The model under review builds one solid part; all positions refer to its coordinate system, in mm. A direction names the side the tool comes from. Round coordinates to 2 decimals unless told otherwise and drop trailing zeros. Order: outer loops, then holes, each group sorted by start corner. A loop starts at its lowest first (then second) coordinate and runs counter-clockwise, first axis right, second up.
Autodesk Fusion 360 part; units mm, degrees
sketch "Sketch1" plane through (0, 0, 0) normal (1, 0, 0) x (0, 0, -1)
  line L0 (-30.1, 40) -> (30.1, 40)
  line L1 (30.1, 40) -> (30.1, -40)
  line L2 (30.1, -40) -> (-30.1, -40)
  line L3 (-30.1, -40) -> (-30.1, 40)
  line L4 (-30.1, 40) -> (30.1, -40) construction
  line L5 (30.1, 40) -> (-30.1, -40) construction
  line L6 (-30.1, 40) -> (-65.1, 40)
  line L7 (-65.1, 40) -> (-65.1, -60)
  line L8 (-65.1, -60) -> (65.1, -60)
  line L9 (65.1, -60) -> (65.1, 40)
  line L10 (65.1, 40) -> (30.1, 40)
  dimension "d1" = 60.2
  dimension "d2" = 80
  dimension "d3" = 35
  dimension "d4" = 20
extrude "Extrude1" add sketch "Sketch1" along normal blind 30 contours L1 L2 L3 L6 L7 L8 L9 L10 makes body 1
sketch "Sketch2" plane through (0, 0, 0) normal (-1, 0, 0) x (0, 0, 1)
  line L0 (-30.1, 40) -> (-65.1, 40)
  line L1 (-65.1, 40) -> (-65.1, -60)
  line L2 (-65.1, -60) -> (65.1, -60)
  line L3 (65.1, -60) -> (65.1, 40)
  line L4 (65.1, 40) -> (30.1, 40)
  line L5 (30.1, 40) -> (30.1, -40)
  line L6 (30.1, -40) -> (-30.1, -40)
  line L7 (-30.1, -40) -> (-30.1, 40)
  line L8 (-47.6, 40) -> (-47.6, -60) construction
  circle A0 centre (-47.6, -0.3557) radius 10.5
  circle A1 centre (-47.6, -40.3557) radius 10.5
  line L9 (0, 0) -> (0, -40) construction
  circle A2 centre (-47.6, -0.3557) radius 4.25
  circle A3 centre (-47.6, -40.3557) radius 4.25
  circle A4 centre (47.6, -0.3557) radius 10.5
  circle A5 centre (47.6, -0.3557) radius 4.25
  circle A6 centre (47.6, -40.3557) radius 4.25
  circle A7 centre (47.6, -40.3557) radius 10.5
  dimension "d8" = 21
  dimension "d11" = 19.6443
  dimension "d12" = 8.5
  dimension "d13" = 8.5
  dimension "d14" = 40
chamfer "Chamfer2" distance 15 angle 45 2 edges at (15, 40, 65.1) (15, 40, -65.1) on bodies 1
chamfer "Chamfer1" distance 15 angle 45 2 edges at (30, -10, 65.1) (30, -10, -65.1) on bodies 1
extrude "Extrude2" cut sketch "Sketch2" against normal blind 60 contours A0 | A1 | A2 | A3 | A4 | A5 | A6 | A7 bodies 1
extrude "Extrude3" add sketch "Sketch2" against normal blind 20 contours A0 | A1 | A4 | A7 bodies 1
sketch "Sketch3" plane through (0, -40, 0) normal (0, 1, 0) x (-1, 0, 0)
  line L0 (0, -30.1) -> (0, 30.1)
  line L1 (0, 30.1) -> (-30, 30.1)
  line L2 (-30, 30.1) -> (-30, -30.1)
  line L3 (-30, -30.1) -> (0, -30.1)
  line L4 (0, 0) -> (-30, 0) construction
  line L5 (-15, 0) -> (-15, 15) construction
  circle A0 centre (-15, 15) radius 5
  circle A1 centre (-15, 15) radius 2.7
  circle A2 centre (-15, -15) radius 5
  circle A3 centre (-15, -15) radius 2.7
  dimension "d20" = 15
  dimension "d21" = 10
  dimension "d22" = 5.4
extrude "Extrude4" cut sketch "Sketch3" against normal blind 20 contours A0 | A1 | A2 | A3 bodies 1
extrude "Extrude5" add sketch "Sketch3" against normal blind 16 contours A0 | A2 bodies 1
sketch "Sketch4" plane through (0, 0, 30.1) normal (0, 0, -1) x (-1, 0, 0)
  line L0 (0, -40) -> (0, 40)
  line L1 (0, 40) -> (-30, 40)
  line L2 (-30, 40) -> (-30, -40)
  line L3 (-30, -40) -> (0, -40)
  line L4 (-15, 40) -> (-15, -40) construction
  circle A0 centre (-15, 25) radius 5
  circle A1 centre (-15, -20) radius 5
  circle A2 centre (-15, -20) radius 2.7
  circle A3 centre (-15, 25) radius 2.7
  dimension "d27" = 10
  dimension "d28" = 5.4
  dimension "d29" = 15
  dimension "d30" = 20
extrude "Extrude6" cut sketch "Sketch4" along normal blind 150 and the other way blind 65 contours A0 | A1 | A2 | A3 bodies 1
extrude "Extrude7" add sketch "Sketch4" against normal blind 18 contours A0 bodies 1
extrude "Extrude8" add sketch "Sketch4" against normal blind 7 contours A1 bodies 1
extrude "Extrude9" add sketch "Sketch4" along normal blind 18 from surface at 60.2 contours A0 bodies 1
extrude "Extrude10" add sketch "Sketch4" along normal blind 7 from surface at 60.2 contours A1 bodies 1
chamfer "Chamfer3" distance 0.4 angle 45 10 faces at (13.3333, -0.5675, 51.8447) (13.3333, -40.5675, 51.8447) (12.3134, -45.3333, 14.7312) (12.3134, -45.3333, -15.2688) (13.3333, -40.5675, -43.3553) (13.3333, -0.5675, -43.3553) (12.3034, 24.8654, 42.1) (12.3134, -20.2688, 34.7667) (12.3034, 24.8654, -42.1) (12.3134, -20.2688, -34.7667) on bodies 1
copy_body "Body->Comp1" bodies 1 removing the originals makes body 2 in component "mousepad stand mount"
component "mousepad stand mount" placed x (1, 0, 0) y (0, 1, 0) z (0, 0, 1) at (0, 0, 0)
(1) Clearance check with flat-ended pins moving along their axes: P1, Ø6, axis at x = 15, y = 25, coming from the +Z side; P2, Ø8.5, axis at x = 15, y = 25, coming from the -Z side; P3, Ø8, axis at x = 13.5, z = -13, coming from the -Y side; P4, Ø9, axis at x = 15, y = -20, coming from the -Z side. State where each tip first meets the part, or that it passes through.
(2) We need section D-D (y = 6.5). Give the boundary of the cut face in (x, z), and give its area (3 significant figures).
(3) Tool access review of faces 1 (the cylindrical face through (23.82, 0.11, 37.11)), 2 (the cylindrical face through (10.381, -21.915, 50.904)), 3 (the flat face through (15, 1, 30.1)): name each direction out of +Z, -Z, +X, -X, +Y, -Y from which nothing blocks a thin tool from reaching the whole face with its end or side.
(4) We need section B-B (z = 15). Give the boundary of the cut face in (x, y).
(5) To check wall thickness, follow L1, parallel to Z at x = 3.25, y = 9; L2, parallel to Y at x = 15, z = 54.5; L3, parallel to Y at x = 26.25, z = 51. State the ranges of each line that lie inside material, in increasing order.
(6) We need section A-A (y = -20). Count the separate pieces of the cut face and the enclosed holes in it, and give its area (3 significant figures).
(7) The part is to be moulded in two halves that separate along Y. For faces 4 (the flat face through (0, -43, 1)), 5 (the flat face through (15.1, -23.3, 37.1)), 6 (the flat face through (15, -40, 0)), say which applies: pulls with the +Y half, pulls with the -Y half, needs draft (parallel to the pull), parting line crosses it, or undercut.
(8) We need section C-C (z = -32). Give the boundary of the cut face in (x, y).
Verdict:
1. P1: stops at z = 48
1. P2: stops at z = -48.1
1. P3: stops at y = -60
1. P4: stops at z = -37.1
2. outline: (0, -65.1) - (15, -65.1) - (24.55, -55.55) - (20, -55.55) - (20, -39.65) - (30, -39.65) - (30, -30.1) - (0, -30.1) - close; (0, 30.1) - (30, 30.1) - (30, 39.65) - (20, 39.65) - (20, 55.55) - (24.55, 55.55) - (15, 65.1) - (0, 65.1) - close
2. area: 1,590 mm2
3. face 1: +X
3. face 2: +Z
3. face 3: +X, -X, +Y
4. outline: (0, -60) - (10, -60) - (10, -56) - (11.9, -56) - (12.3, -55.6) - (12.3, -40.4) - (11.9, -40) - (0, -40) - close; (17.7, -55.6) - (18.1, -56) - (20, -56) - (20, -60) - (30, -60) - (30, -40) - (18.1, -40) - (17.7, -40.4) - close
5. L1: z = -65.1 to -30.1, 30.1 to 65.1
5. L2: y = -60 to -25, -15 to 20, 30 to 35.6
5. L3: y = -60 to -50.29, -30.42 to -10.29, 9.58 to 39.1
6. separate pieces: 4
6. enclosed holes: 0
6. area: 1,260 mm2
7. face 4: needs draft
7. face 5: undercut
7. face 6: pulls with the +Y half
8. outline: (0, -60) - (30, -60) - (30, 40) - (0, 40) - close; hole circle Ø5.4 at (15, -20); hole circle Ø5.4 at (15, 25)
